Can you work these out from the model? Positions are in its coordinate system, mm. Face numbers are marked on the shaded views. A direction names the side the tool comes from. Give positions to 0.01 mm unless a question says otherwise; leave off trailing zeros. Write each loop counter-clockwise with the first axis right and the second up, starting at its lowest first coordinate (ties: lowest second). Pieces come first, ordered by that corner, then holes.
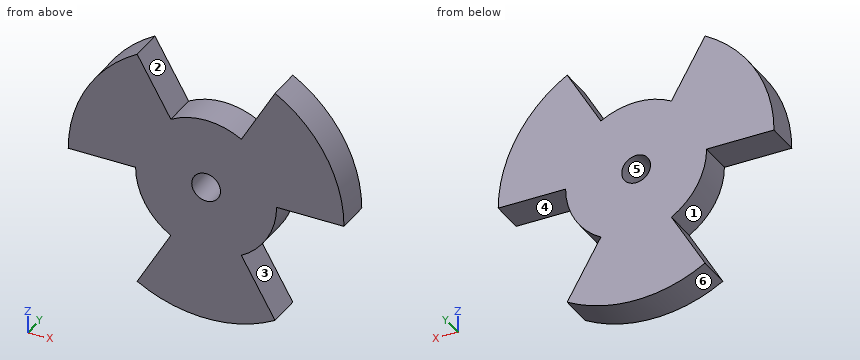
Autodesk Inventor part; units mm, degrees
ref_plane "YZ Plane" through (0, 0, 0) normal (1, 0, 0) x (0, 1, 0)
ref_plane "XZ Plane" through (0, 0, 0) normal (0, 1, 0) x (-1, 0, 0)
ref_plane "XY Plane" through (0, 0, 0) normal (0, 0, 1) x (1, 0, 0)
sketch "Sketch1" plane through (0, 0, 0) normal (0, 1, 0) x (1, 0, 0)
  circle A0 centre (0, 0) radius 25
  arc A1 (24.4487, 42.3463) -> (-24.4487, 42.3463) centre (0, 0) ccw
  line L0 (12.5, 21.6506) -> (24.4487, 42.3463)
  line L1 (-12.5, 21.6506) -> (-24.4487, 42.3463)
  line L2 (0, 0) -> (0, 84.0286) construction
  line L3 (-12.5, -21.6506) -> (-24.4487, -42.3463)
  arc A2 (-48.8973, 0) -> (-24.4487, -42.3463) centre (0, 0) ccw
  line L4 (-25, 0) -> (-48.8973, 0)
  line L5 (25, 0) -> (48.8973, 0)
  arc A3 (24.4487, -42.3463) -> (48.8973, 0) centre (0, 0) ccw
  line L6 (12.5, -21.6506) -> (24.4487, -42.3463)
  point P0 (25, 0)
  dimension "d0" = 50
  dimension "d1" = 60
  dimension "d2" = 30
  dimension "d5" = 360
extrude "Extrusion1" add sketch "Sketch1" along normal blind 12
sketch "Sketch4" plane through (0, 0, 0) normal (0, -1, 0) x (1, 0, 0)
  circle A0 centre (0, 0) radius 7.9289
  point P0 (0, 0)
hole "Hole2" at (0, 0, 0) direction (0, 1, 0) diameter 10.2 depth 12
properties part number "rotor"
1) Suppose I cut it at A-A on x = 0. Write out the boundary of the cut face in (y, z), plus the area to 3 significant figures.
Values follow:
outline: (0, -48.9) - (12, -48.9) - (12, -5.1) - (0, -5.1) - close; (0, 5.1) - (12, 5.1) - (12, 25) - (0, 25) - close
area: 764 mm2
2) Suppose I cut it at B-B on z = 33.5. Write out the boundary of the cut face in (x, y), plus the area to 3 significant figures.
Values follow:
outline: (-35.62, 0) - (-19.34, 0) - (-19.34, 12) - (-35.62, 12) - close; (19.34, 0) - (35.62, 0) - (35.62, 12) - (19.34, 12) - close
area: 391 mm2
3) If we mould it in two halves opening along X, with no side actions, what happens to the marked faces 4, 5 and 6? For each: +X half, -X half, draft (parallel to the pull), parting line (faces both ways), or undercut.
Values follow:
face 4: draft
face 5: undercut
face 6: parting line
4) For the marked faces 1, 2 and 3, which set-ups out of +Z, -Z, +X, -X, +Y, -Y let a thin tool reach every point of the face, with its end or its side?
Values follow:
face 1: -X, +Y, -Y
face 2: +Z, +Y, -Y
face 3: +X, +Y, -Y
5) Suppose I cut it at D-D on x = 34.5. Write out the boundary of the cut face in (y, z), plus the area to 3 significant figures.
Values follow:
outline: (0, 0) - (12, 0) - (12, 34.65) - (0, 34.65) - close
area: 416 mm2
6) Suppose I cut it at C-C on y = 2.25. Write out the boundary of the cut face in (x, z), plus the area to 3 significant figures.
Values follow:
outline: (-48.9, 0) - (-25, 0) arc R25 ccw to (-12.5, -21.65) - (-24.45, -42.35) arc R48.9 ccw to (24.45, -42.35) - (12.5, -21.65) arc R25 ccw to (25, 0) - (48.9, 0) arc R48.9 ccw to (24.45, 42.35) - (12.5, 21.65) arc R25 ccw to (-12.5, 21.65) - (-24.45, 42.35) arc R48.9 ccw to start; hole circle Ø10.2 at (0, 0)
area: 4,660 mm2
7) For pin 1 Ø3 at (x, y) = (33.5, 7) entering from -Z; pin 2 Ø6 at (y, z) = (10.5, 30.5) entering from -X; pin 3 Ø4 at (x, y) = (-7, 8.5) entering from -Z; pin 4 Ø9 at (x, z) = (0, 0) entering from -Y, each with a flat end and sliding along its axis, tell me the tip position at first contact or that it passes through.
Values follow:
pin 1: stops at z = 0
pin 2: stops at x = -40.43
pin 3: stops at z = -48.64
pin 4: passes through
8) Please list where these lines run through material, in increasing order: L1, parallel to Z at x = 0, y = 4.5; L2, parallel to X at y = 7, z = 36; L3, parallel to Z at x = -1, y = 3.5.
Values follow:
L1: z = -48.9 to -5.1, 5.1 to 25
L2: x = -33.09 to -20.78, 20.78 to 33.09
L3: z = -48.89 to -5, 5 to 24.98
